Here's how the part is built. I have some questions about the finished solid (model axes, mm). A direction names the side the tool comes from. Round coordinates to 2 decimals unless told otherwise and drop trailing zeros. Loops run counter-clockwise (first coordinate to the right, second up) from the corner with the lowest first, then second, coordinate; pieces in that order, holes last. Notation, with made-up numbers: M 46,-14 L 100,-14 A24 cw 100,22 Z; hole C 39,-28.5 d11. An arc over 180 degrees is marked long. Answer as a JSON object with one key per item and string values.
from build123d import *

# Parameters (mm, degrees)
BOSS_EXTRUDE1_DEPTH = 4
SKETCH2_R           = 1.5
CUT_EXTRUDE2_DEPTH  = 4


with BuildPart() as part:
    # Sketch1 → Boss-Extrude1 (new body)
    with BuildSketch(Plane(origin=(0, 0, 0), x_dir=(1, 0, 0), z_dir=(0, 1, 0))):
        Polygon((55, 10), (-55, 10), (-55, 3.5), (-51, 3.5), (-51, -3.5), (-55, -3.5), (-55, -10), (55, -10), (55, -3.5), (51, -3.5), (51, 3.5), (55, 3.5), align=None)
    extrude(amount=BOSS_EXTRUDE1_DEPTH)

    # Sketch2 → Cut-Extrude2 (cut)
    with BuildSketch(Plane.XZ):
        with BuildLine():
            ThreePointArc((-23.5, 0), (-23.939339828, -1.060660172), (-25, -1.5))
            Line((-25, -1.5), (25, -1.5))
            ThreePointArc((25, -1.5), (23.5, 0), (25, 1.5))
            Line((25, 1.5), (-25, 1.5))
            ThreePointArc((-25, 1.5), (-23.939339828, 1.060660172), (-23.5, 0))
        make_face()
        with Locations((-25, 0)):
            Circle(SKETCH2_R)
        with Locations((25, 0)):
            Circle(SKETCH2_R)
    extrude(amount=-CUT_EXTRUDE2_DEPTH, mode=Mode.SUBTRACT)


solid = part.part
Item 1: I'm going to push flat-ended pins straight in: pin 1 Ø1.2 at (y, z) = (1.5, 1) entering from -X; pin 2 Ø1.2 at (y, z) = (2.5, 0.5) entering from +X. Where does each tip first touch, or does it pass through?
Resolved:
{"pin 1": "x = -51", "pin 2": "x = 51"}
Item 2: If we mould it in two halves opening along Z, with no side actions, what happens to faces 1 (the face through (53, 2, 3.5)), 2 (the face through (55, 2, 7)), 3 (the face through (1, 2, -10))? For each: pulls with the +Z half, pulls with the -Z half, needs draft (parallel to the pull), parting line crosses it, or undercut.
Resolved:
{"face 1": "undercut", "face 2": "needs draft", "face 3": "pulls with the -Z half"}
Item 3: On a 3-axis mill with a long thin cutter (end or side, diameter ignored), from which of +Z, -Z, +X, -X, +Y, -Y can I reach the whole of each face in a straight line? I mean faces 4 (the face through (53, 2, -3.5)), 5 (the face through (-26.5, 2, 0)), 6 (the face through (-51, 2, 0)). Say none if no direction works.
Resolved:
{"face 4": "+X, +Y, -Y", "face 5": "+Y, -Y", "face 6": "-X, +Y, -Y"}
Item 4: I want a section at C-C, the plane y = 1.6. Please give me the cut outline in (x, z).
Resolved:
{"outline": "M -55,-10 L 55,-10 L 55,-3.5 L 51,-3.5 L 51,3.5 L 55,3.5 L 55,10 L -55,10 L -55,3.5 L -51,3.5 L -51,-3.5 L -55,-3.5 Z; hole M -25,-1.5 L 25,-1.5 A1.5 ccw 25,1.5 L -25,1.5 A1.5 ccw Z"}
Item 5: I want a section at A-A, the plane x = 16. Please give me the cut outline in (y, z).
Resolved:
{"outline": "M 0,-10 L 4,-10 L 4,-1.5 L 0,-1.5 Z; M 0,1.5 L 4,1.5 L 4,10 L 0,10 Z"}
Item 6: I want a section at B-B, the plane z = 0. Please give me the cut outline in (x, y), then the cut area to 3 significant figures.
Resolved:
{"outline": "M -51,0 L -26.5,0 L -26.5,4 L -51,4 Z; M 26.5,0 L 51,0 L 51,4 L 26.5,4 Z", "area": "196 mm²"}
Item 7: Please list where these lines run through material, in increasing order: probe 1 along Z at (x, y) = (0.5, 1.7); probe 2 along X at (y, z) = (2.6, 2.25); probe 3 along X at (y, z) = (1.55, 0.5). Write a range as from..to.
Resolved:
{"probe 1": "-10..-1.5, 1.5..10", "probe 2": "-51..51", "probe 3": "-51..-26.41, 26.41..51"}
